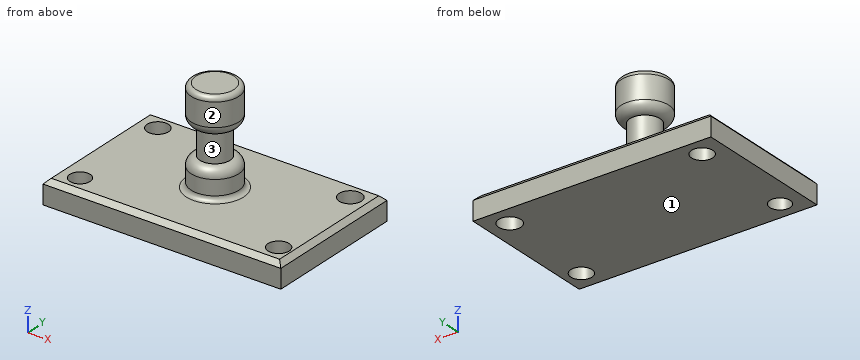
from build123d import *

# Parameters (mm, degrees)
F0_W     = 127
F0_H     = 76.2
F1_DEPTH = 12.7
F2_R     = 5.9427105428
F2_R_2   = 5.6670127921
F2_R_3   = 5.7023762048
F2_R_4   = 5.4269658504
F3_DEPTH = 12.7
F4_W     = 12.7
F4_H     = 50.8
F6_W     = 9.3170334585
F6_H     = 15.1401739568
F8_R     = 2.54
F9_SIZE  = 2.54


# Not quite as in the source:
# - a fillet or chamfer that OpenCascade refuses, or shapes differently, is made with other operations: its cross-section is extruded or revolved along the edge and cut away or added


with BuildPart() as f1:
    # F0 (on Top) → F1 (new body)
    with BuildSketch(Plane.XY):
        Rectangle(F0_W, F0_H)
    extrude(amount=F1_DEPTH)

    # F2 (on Top) → F3 (cut)
    with BuildSketch(Plane.XY):
        with Locations((52.0129092038, 27.1925590932)):
            Circle(F2_R)
        with Locations((54.2030967772, -27.1966736764)):
            Circle(F2_R_2)
        with Locations((-51.2907654047, 27.9071591794)):
            Circle(F2_R_3)
        with Locations((-51.2907616794, -27.9425289482)):
            Circle(F2_R_4)
    extrude(amount=F3_DEPTH, mode=Mode.SUBTRACT)

    # F4 (on Front) → F5 (revolve)
    with BuildSketch(Plane.XZ):
        with Locations((6.35, 38.1)):
            Rectangle(F4_W, F4_H)
    revolve(axis=Axis((0, 0, 38.1), (0, 0, 1)))

    # F6 (on Front) → F7 (revolve, cut)
    with BuildSketch(Plane.XZ):
        with Locations((12.6875618007, 35.8667755499)):
            Rectangle(F6_W, F6_H)
    revolve(axis=Axis((0, 0, 12.7), (0, 0, 1)), mode=Mode.SUBTRACT)

    # F8
    f8_edges = [f1.edges().sort_by_distance(p)[0] for p in [
        (-12.7, 0, 63.5),
        (-12.7, 0, 12.7),
    ]]
    fillet(f8_edges, radius=F8_R)

    # F9
    f9_edges = [f1.edges().sort_by_distance(p)[0] for p in [
        (0, -38.1, 12.7),
        (0, 38.1, 12.7),
        (63.5, 0, 12.7),
        (-63.5, 0, 12.7),
    ]]
    chamfer(f9_edges, length=F9_SIZE)

    # F10: fillet of radius 5.08 on 2 edges, made by hand

    # F10_s1 → F10_t2 (revolve, cut)
    with BuildSketch(Plane.XZ):
        with BuildLine():
            ThreePointArc((8.0290450715, 43.4368625283), (11.3539221311, 45.0559189466), (12.7, 48.5003674537))
            Line((12.7, 48.5003674537), (12.7, 43.4368625283))
            Line((12.7, 43.4368625283), (8.0290450715, 43.4368625283))
        make_face()
    revolve(axis=Axis((0, 0, 43.4368625283), (0, 0, 1)), mode=Mode.SUBTRACT)

    # F10_s3 → F10_t4 (revolve, cut)
    with BuildSketch(Plane.XZ):
        with BuildLine():
            ThreePointArc((12.7, 23.2331836462), (11.3539221311, 26.6776321533), (8.0290450715, 28.2966885716))
            Line((8.0290450715, 28.2966885716), (12.7, 28.2966885716))
            Line((12.7, 28.2966885716), (12.7, 23.2331836462))
        make_face()
    revolve(axis=Axis((0, 0, 28.2966885716), (0, 0, 1)), mode=Mode.SUBTRACT)


solid = f1.part
CAD build for the part. Positions are in the model's coordinates, mm. Face numbers are marked on the shaded views. A direction names the side the tool comes from. Give positions to 0.01 mm unless a question says otherwise; leave off trailing zeros. Write each loop counter-clockwise with the first axis right and the second up, starting at its lowest first coordinate (ties: lowest second). Pieces come first, ordered by that corner, then holes. Notation, with made-up numbers: (7.25, -32.75) - (66.25, -32.75) arc R20 ccw to (66.25, -25.75) - close; hole circle Ø7 at (29, 17.25). An arc over 180 degrees is marked (long way). Answer as CSV lines item,"result".
Q1. 3-axis set-ups, long thin cutter, end or side, ignore diameter. For the marked faces 1, 2 and 3: which of +Z, -Z, +X, -X, +Y, -Y reach the whole face in a straight line?
Result set:
face 1,"-Z, +X, -X, +Y, -Y"
face 2,"+Z"
face 3,"none"
Q2. Band-saw the part on A-A (x = 0). Give the cut face in (y, z).
Result set:
outline,"(-38.1, 0) - (38.1, 0) - (38.1, 10.16) - (35.56, 12.7) - (15.24, 12.7) arc R2.54 cw to (12.7, 15.24) - (12.7, 23.23) arc R5.08 ccw to (8.03, 28.3) - (8.03, 43.44) arc R5.08 ccw to (12.7, 48.5) - (12.7, 60.96) arc R2.54 ccw to (10.16, 63.5) - (-10.16, 63.5) arc R2.54 ccw to (-12.7, 60.96) - (-12.7, 48.5) arc R5.08 ccw to (-8.03, 43.44) - (-8.03, 28.3) arc R5.08 ccw to (-12.7, 23.23) - (-12.7, 15.24) arc R2.54 cw to (-15.24, 12.7) - (-35.56, 12.7) - (-38.1, 10.16) - close"
Q3. Band-saw the part on C-C (y = 0). Give the cut face in (x, z), and give its area (3 significant figures).
Result set:
outline,"(-63.5, 0) - (63.5, 0) - (63.5, 10.16) - (60.96, 12.7) - (15.24, 12.7) arc R2.54 cw to (12.7, 15.24) - (12.7, 23.23) arc R5.08 ccw to (8.03, 28.3) - (8.03, 43.44) arc R5.08 ccw to (12.7, 48.5) - (12.7, 60.96) arc R2.54 ccw to (10.16, 63.5) - (-10.16, 63.5) arc R2.54 ccw to (-12.7, 60.96) - (-12.7, 48.5) arc R5.08 ccw to (-8.03, 43.44) - (-8.03, 28.3) arc R5.08 ccw to (-12.7, 23.23) - (-12.7, 15.24) arc R2.54 cw to (-15.24, 12.7) - (-60.96, 12.7) - (-63.5, 10.16) - close"
area,"2,730 mm²"
Q4. Flat gauge pins, fed straight in: pin 1 Ø1 at (y, z) = (-6.5, 51.5) entering from -X; pin 2 Ø6 at (x, y) = (7, -30.5) entering from -Z; pin 3 Ø1.5 at (x, z) = (1.5, 15.5) entering from +Y; pin 4 Ø4 at (x, y) = (45.5, -17) entering from +Z. Where does each tip first touch, or does it go through?
Result set:
pin 1,"x = -11.19"
pin 2,"z = 0"
pin 3,"y = 12.68"
pin 4,"z = 12.7"
Q5. Band-saw the part on D-D (z = 39.5). Give the cut face in (x, y), and give its area (3 significant figures).
Result set:
outline,"circle Ø16.06 at (0, 0)"
area,"203 mm²"
Q6. Band-saw the part on B-B (z = 8). Give the cut face in (x, y).
Result set:
outline,"(-63.5, -38.1) - (63.5, -38.1) - (63.5, 38.1) - (-63.5, 38.1) - close; hole circle Ø11.4 at (-51.29, 27.91); hole circle Ø10.85 at (-51.29, -27.94); hole circle Ø11.89 at (52.01, 27.19); hole circle Ø11.33 at (54.2, -27.2)"
Q7. Drill centre lines: line 1 (Z direction, x = 22.5, y = -13); line 2 (X direction, y = 0.5, z = 55.5); line 3 (Z direction, x = 10, y = 5). Where is each one in solid material? Low to high. Write a range as from..to.
Result set:
line 1,"0..12.7"
line 2,"-12.69..12.69"
line 3,"0..26.86, 44.88..63.29"
